from build123d import *

# Parameters (mm, degrees)
F0_W     = 20
F0_H     = 15.6083446927
F0_W_2   = 3
F0_H_2   = 3
F0_R     = 1.25
F0_R_2   = 3.25
F1_DEPTH = 6
F2_R     = 1.25
F3_DEPTH = 5.6
F4_W     = 20
F4_H     = 15.6083446927
F4_W_2   = 19.2
F4_H_2   = 14.8083446927
F5_DEPTH = 3
F7_START = -0.6
F6_R     = 1.4
F7_DEPTH = 4.8
F8_R     = 1


with BuildPart() as f1:
    # F0 (on Top) → F1 (new body)
    with BuildSketch(Plane.XY):
        with Locations((1.4342954904, -0.0335501973)):
            Rectangle(F0_W, F0_H)
        with Locations((-3.3330191961, -3.9553961381)):
            Rectangle(F0_W_2, F0_H_2, mode=Mode.SUBTRACT)
        with Locations((-4.2153447866, 4.6489532106)):
            Circle(F0_R, mode=Mode.SUBTRACT)
        with Locations((3.6709753331, 0)):
            Circle(F0_R_2, mode=Mode.SUBTRACT)
    extrude(amount=F1_DEPTH)

    # F2 (on face) → F3 (cut)
    with BuildSketch(Plane(origin=(0, 0, 0), x_dir=(1, 0, 0), z_dir=(0, 0, -1))):
        with Locations((8.7077384815, 5.1523931324)):
            Circle(F2_R)
    extrude(amount=-F3_DEPTH, mode=Mode.SUBTRACT)

    # F4 (on face) → F5 (cut)
    with BuildSketch(Plane(origin=(0, 0, 0), x_dir=(1, 0, 0), z_dir=(0, 0, -1))):
        with Locations((1.4342954904, 0.0335501973)):
            Rectangle(F4_W, F4_H)
        with Locations((1.4342954904, 0.0335501973)):
            Rectangle(F4_W_2, F4_H_2, mode=Mode.SUBTRACT)
    extrude(amount=-F5_DEPTH, mode=Mode.SUBTRACT)

    # F6 (on face) → F7 (cut)
    with BuildSketch(Plane(origin=(0, 0, 0), x_dir=(1, 0, 0), z_dir=(0, 0, -1)).offset(F7_START)):
        with Locations((8.1054680049, -4.4064032845)):
            Circle(F6_R)
    extrude(amount=-F7_DEPTH, mode=Mode.SUBTRACT)

    # F8
    f8_edges = [f1.edges().sort_by_distance(p)[0] for p in [
        (11.034295, 7.370622, 1.5),
        (-8.165705, 7.370622, 1.5),
        (-8.165705, -7.437723, 1.5),
        (11.034295, -7.437723, 1.5),
    ]]
    fillet(f8_edges, radius=F8_R)


solid = f1.part
Geometry: final body of the model. Coordinates: model frame, mm. A direction names the side the tool comes from. Round coordinates to 2 decimals unless told otherwise and drop trailing zeros. Write each loop counter-clockwise with the first axis right and the second up, starting at its lowest first coordinate (ties: lowest second). Pieces come first, ordered by that corner, then holes. Notation, with made-up numbers: M 24.5,46.25 L 29.5,46.25 A19 ccw 29.5,57.25 Z; hole C 5.5,53.25 d3. An arc over 180 degrees is marked long. Write item = value, one per line.
Item 1: Section query C-C on x = -6.5. Return loops of the section in (y, z), then the cut area to 4 significant figures.
Findings:
outline = M -7.84,3 L -7.44,3 L -7.44,0 L 7.37,0 L 7.37,3 L 7.77,3 L 7.77,6 L -7.84,6 Z
area = 91.25 mm^2
Item 2: Section query B-B on x = 3.75. Return loops of the section in (y, z), then the cut area to 3 significant figures.
Findings:
outline = M -7.84,3 L -7.44,3 L -7.44,0 L -3.25,0 L -3.25,6 L -7.84,6 Z; M 3.25,0 L 7.37,0 L 7.37,3 L 7.77,3 L 7.77,6 L 3.25,6 Z
area = 52.3 mm^2
Item 3: Section query A-A on y = 0. Return loops of the section in (x, z).
Findings:
outline = M -8.57,3 L -8.17,3 L -8.17,0 L 0.42,0 L 0.42,6 L -8.57,6 Z; M 6.92,0 L 11.03,0 L 11.03,3 L 11.43,3 L 11.43,6 L 6.92,6 Z
Item 4: Material intervals for line 1 along Y through (x, z) = (-4.25, 1.6); line 2 along X through (y, z) = (-3.5, 3.35); line 3 along X through (y, z) = (-5, 1.85), sorted ascending. Write a range as [from, to].
Findings:
line_1 = [-7.44, -5.46], [-2.46, 3.4], [5.9, 7.37]
line_2 = [-8.57, -4.83], [-1.83, 11.43]
line_3 = [-8.17, -4.83], [-1.83, 7.47], [9.95, 11.03]
Item 5: Section query D-D on z = 1.2. Return loops of the section in (x, y).
Findings:
outline = M -8.17,-6.44 A1 ccw -7.17,-7.44 L 10.03,-7.44 A1 ccw 11.03,-6.44 L 11.03,6.37 A1 ccw 10.03,7.37 L -7.17,7.37 A1 ccw -8.17,6.37 Z; hole C -4.22,4.65 d2.5; hole M -4.83,-5.46 L -1.83,-5.46 L -1.83,-2.46 L -4.83,-2.46 Z; hole C 3.67,0 d6.5; hole C 8.11,4.41 d2.8; hole C 8.71,-5.15 d2.5
Item 6: Pull-direction query (Z, two-part tool) for faces 6 (the face through (-1, 0, 0)), 7 (the face through (6.707, 4.345, 2.966)), 8 (the face through (1, 7.771, 4)); classes: pulls with the +Z half, pulls with the -Z half, needs draft (parallel to the pull), parting line crosses it, or undercut.
Findings:
face_6 = pulls with the -Z half
face_7 = undercut
face_8 = needs draft
Item 7: Pin query (flat end, axial travel): P1, Ø0.9, axis at x = -2.5, z = 2, coming from the -Y side; P2, Ø1, axis at y = -0.5, z = 2, coming from the -X side; P3, Ø6, axis at x = 3.67, y = 0, coming from the +Z side; P4, Ø0.9, axis at x = 2, z = 1, coming from the +Y side. Return the tip coordinate at first contact, or that it passes through.
Findings:
P1 = -7.44
P2 = -8.17
P3 = through
P4 = 7.37
Item 8: Access query for faces 1 (the face through (9, -5, 5.6)), 2 (the face through (-7.86, 7.09, 1.52)), 3 (the face through (8, 4, 0.6)), 4 (the face through (-4.833, -4, 3)), 5 (the face through (10.749, -7.137, 1.521)). Directions: +Z, -Z, +X, -X, +Y, -Y. A direction counts if a zero-diameter tool reaches every point of the face in a straight line with its end or side. Return the directions, or none.
Findings:
face_1 = -Z
face_2 = -Z, -X, +Y
face_3 = none
face_4 = +Z, -Z
face_5 = -Z, +X, -Y
